Check sheet for the modelled part. Datum: model origin and axes. Units: mm. Face numbers are marked on the shaded views. A direction names the side the tool comes from. Give positions to 0.01 mm unless a question says otherwise; leave off trailing zeros. Loops run counter-clockwise (first coordinate to the right, second up) from the corner with the lowest first, then second, coordinate; pieces in that order, holes last. Notation, with made-up numbers: M 57.5,-36 L 65.5,-36 A17 cw 65.5,-30 Z; hole C -5.5,7 d11. An arc over 180 degrees is marked long. Put each result on its own line as item: value. Start each with the question number.
```python
from build123d import *

# Parameters (mm, degrees)
F0_R      = 30
F0_R_2    = 20
F1_DEPTH  = 60
F2_R      = 20
F2_R_2    = 9.9351128524
F3_DEPTH  = 15
F5_DEPTH  = 45
F6_SIZE2  = 24.99999
F6_SIZE   = 44.99999
F7_R      = 20
F8_DEPTH  = 15
F10_DEPTH = 30
F11_R     = 8
F12_DEPTH = 15


# Not quite as in the source:
# - a fillet or chamfer is up to 0.001 mm smaller than in the source, because OpenCascade refuses the exact size


with BuildPart() as f1:
    # F0 (on Top) → F1 (new body)
    with BuildSketch(Plane.XY):
        Circle(F0_R)
        Circle(F0_R_2, mode=Mode.SUBTRACT)
    extrude(amount=F1_DEPTH)

    # F2 (on Top) → F3 (join)
    with BuildSketch(Plane.XY):
        with BuildLine():
            Line((16.7213538347, -24.9077563409), (75, -24.9077563409))
            ThreePointArc((75, -24.9077563409), (99.9077563409, 0), (75, 24.9077563409))
            Line((75, 24.9077563409), (16.7213538347, 24.9077563409))
            ThreePointArc((16.7213538347, 24.9077563409), (-30, 0), (16.7213538347, -24.9077563409))
        make_face()
        Circle(F2_R, mode=Mode.SUBTRACT)
        with Locations((75, 0)):
            Circle(F2_R_2, mode=Mode.SUBTRACT)
    extrude(amount=F3_DEPTH)

    # F4 (on face) → F5 (join, through all)
    with BuildSketch(Plane.XY.offset(15)):
        with BuildLine():
            Line((54.5803989155, 5), (29.5803989155, 5))
            ThreePointArc((29.5803989155, 5), (30, 0), (29.5803989155, -5))
            Line((29.5803989155, -5), (54.5803989155, -5))
            Line((54.5803989155, -5), (54.5803989155, 5))
        make_face()
    extrude(amount=F5_DEPTH)

    # F6 (size 45 and 25 in the source; OpenCascade refuses exactly that, so slightly less here)
    f6_edges = [f1.edges().sort_by_distance(p)[0] for p in [
        (54.580399, 0, 60),
    ]]
    f6_side = f1.faces().sort_by_distance((54.580399, 0, 37.5))[0]
    chamfer(f6_edges, length=F6_SIZE, length2=F6_SIZE2, reference=f6_side)

    # F7 (on face) → F8 (join)
    with BuildSketch(Plane.XY.offset(15)):
        with BuildLine():
            Line((29.5803989155, -5), (29.5803989155, 5))
            ThreePointArc((29.5803989155, 5), (19.364916731, 22.9128784748), (0, 30))
            ThreePointArc((0, 30), (-30, 0), (0, -30))
            ThreePointArc((0, -30), (19.364916731, -22.9128784748), (29.5803989155, -5))
        make_face()
        Circle(F7_R, mode=Mode.SUBTRACT)
        with BuildLine():
            ThreePointArc((0, -30), (-30, 0), (0, 30))
            Line((0, 30), (-75, 30))
            Line((-75, 30), (-75, -30))
            Line((-75, -30), (0, -30))
        make_face()
    extrude(amount=F8_DEPTH)

    # F9 (on face) → F10 (join, through all)
    with BuildSketch(Plane.XY.offset(30)):
        with BuildLine():
            Line((-60, 30), (-75, 30))
            Line((-75, 30), (-75, -30))
            Line((-75, -30), (-60, -30))
            Line((-60, -30), (-60, -5))
            Line((-60, -5), (-29.5803989155, -5))
            ThreePointArc((-29.5803989155, -5), (-30, 0), (-29.5803989155, 5))
            Line((-29.5803989155, 5), (-60, 5))
            Line((-60, 5), (-60, 30))
        make_face()
    extrude(amount=F10_DEPTH)

    # F11 (on face) → F12 (cut, through all)
    with BuildSketch(Plane(origin=(-75, 0, 0), x_dir=(0, -1, 0), z_dir=(-1, 0, 0))):
        with Locations((17.5, 45)):
            Circle(F11_R)
        with Locations((-17.5, 45)):
            Circle(F11_R)
    extrude(amount=-F12_DEPTH, mode=Mode.SUBTRACT)


solid = f1.part
```
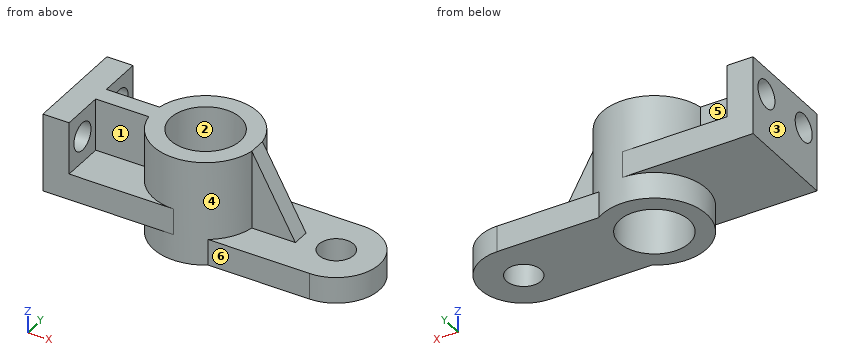
Q1. Thickness scan on line 1 along Z through (x, y) = (-70.5, -17.5); line 2 along X through (y, z) = (-8.5, 56); line 3 along X through (y, z) = (11.5, 52.5). Record the ranges inside material, lowest first. Write a range as [from, to].
Q2. Mould release check, pull along Y, two halves, no side actions. Record for the marked faces 1, 2 and 3: pulls with the +Y half, pulls with the -Y half, needs draft (parallel to the pull), parting line crosses it, or undercut.
Q3. Section check C-C, the plane z = 11. Record the cut outline in (x, y).
Q4. Depth check by flat-ended pin: P1, Ø7.5, axis at x = 44, z = 6.5, coming from the +Y side; P2, Ø3, axis at x = 81.5, y = -19, coming from the -Z side; P3, Ø18.5, axis at y = -17.5, z = 45, coming from the +X side; P4, Ø15, axis at x = 43.5, y = -6.5, coming from the +Z side. Enter the tip coordinate at first touch or a pass-through.
Q5. Section check D-D, the plane x = 24. Record the cut outline in (y, z), then the cut area to 3 significant figures.
Q6. Section check A-A, the plane z = 45. Record the cut outline in (x, y), then the cut area to 3 significant figures.
Q7. Section check B-B, the plane y = 17.5. Record the cut outline in (x, z).
Q8. Access from +Z, -Z, +X, -X, +Y, -Y to the whole of each face (thin tool, end or side, straight path). Record for the marked faces 4, 5 and 6.
Found:
1. line 1: z = [15, 37], [53, 60]
1. line 2: x = [-75, -60], [-28.77, -18.1], [18.1, 28.77]
1. line 3: x = [-75, -60], [-27.71, -16.36], [16.36, 27.71]
2. face 1: pulls with the -Y half
2. face 2: undercut
2. face 3: needs draft
3. outline: M 16.72,-24.91 L 75,-24.91 A24.91 ccw 75,24.91 L 16.72,24.91 A30 ccw long Z; hole C 0,0 d40; hole C 75,0 d19.87
4. P1: stops at y = 24.91
4. P2: stops at z = 0
4. P3: stops at x = 28.84
4. P4: stops at z = 48.17
5. outline: M -24.91,0 L 24.91,0 L 24.91,15 L 18,15 L 18,60 L -18,60 L -18,15 L -24.91,15 Z
5. area: 2,370 mm^2
6. outline: M -75,-30 L -60,-30 L -60,-25.5 L -75,-25.5 Z; M -75,-9.5 L -60,-9.5 L -60,-5 L -29.58,-5 A30 ccw 29.58,-5 L 37.91,-5 L 37.91,5 L 29.58,5 A30 ccw -29.58,5 L -60,5 L -60,9.5 L -75,9.5 Z; M -75,25.5 L -60,25.5 L -60,30 L -75,30 Z; hole C 0,0 d40
6. area: 2,370 mm^2
7. outline: M -75,15 L -24.37,15 L -24.37,0 L -9.68,0 L -9.68,60 L -24.37,60 L -24.37,30 L -60,30 L -60,37 L -75,37 Z; M -75,53 L -60,53 L -60,60 L -75,60 Z; M 9.68,0 L 92.72,0 L 92.72,15 L 24.37,15 L 24.37,60 L 9.68,60 Z
8. face 4: none
8. face 5: +Z, +Y
8. face 6: +Z, -Z, +X, -Y
